For this review, take the finished solid that the model builds, in its own axes (mm). A direction names the side the tool comes from. Give positions to 0.01 mm unless a question says otherwise; leave off trailing zeros. Write each loop counter-clockwise with the first axis right and the second up, starting at its lowest first coordinate (ties: lowest second). Pieces come first, ordered by that corner, then holes. Notation, with made-up numbers: (21, 28) -> (26, 28) arc R9 ccw to (26, 32) -> close; hole circle Ø1 at (9, -30). An arc over 180 degrees is marked (long way). Write item = value, one per line.
```python
from build123d import *

# Parameters (mm, degrees)
BOSS_EXTRUDE1_DEPTH      = 25
BOSS_EXTRUDE1_DEPTH_BACK = 32
SKETCH2_R                = 45
CUT_EXTRUDE1_DEPTH       = 45
CUT_EXTRUDE2_REACH       = 139.165
CUT_EXTRUDE2_END_RADIUS  = 45
SKETCH3_R                = 16
CIRPATTERN1_COUNT        = 6
CHAMFER2_SIZE            = 2
FILLET1_R                = 2


with BuildPart() as part:
    # Sketch1 → Boss-Extrude1 (new, two sides: drawn at the far end of the back side and taken through both)
    with BuildSketch(Plane.XY.offset(-BOSS_EXTRUDE1_DEPTH_BACK)):
        Polygon((0, 61.199128534), (-53, 30.599564267), (-53, -30.599564267), (0, -61.199128534), (53, -30.599564267), (53, 30.599564267), align=None)
    extrude(amount=BOSS_EXTRUDE1_DEPTH + BOSS_EXTRUDE1_DEPTH_BACK)

    # Sketch2 → Cut-Extrude1 (cut)
    with BuildSketch(Plane.XY.offset(25)):
        Circle(SKETCH2_R)
    extrude(amount=-CUT_EXTRUDE1_DEPTH, mode=Mode.SUBTRACT)

    # Cut-Extrude2: up to this cylinder (the profile starts outside it)
    cut_extrude2_end = Plane(origin=(0, 0, 0), z_dir=(0, 0, 1)) * Cylinder(CUT_EXTRUDE2_END_RADIUS, 369.33, mode=Mode.PRIVATE)
    # Sketch3 → Cut-Extrude2 (cut, up to the surface)
    with BuildSketch(Plane(origin=(26.5, -45.899346401, 0), x_dir=(0.8660254037844387, 0.4999999999999999, 0), z_dir=(0.4999999999999999, -0.8660254037844387, 0)), mode=Mode.PRIVATE) as cut_extrude2_sk1:
        Circle(SKETCH3_R)
    cut_extrude2_tool1 = extrude(cut_extrude2_sk1.sketch, amount=-CUT_EXTRUDE2_REACH, mode=Mode.PRIVATE) - cut_extrude2_end
    cut_extrude2 = cut_extrude2_tool1.solids().sort_by_distance((26.5, -45.899346, 0))[0]
    add(cut_extrude2, mode=Mode.SUBTRACT)

    # CirPattern1: Cut-Extrude2 ×6 about axis
    cirpattern1_axis = Axis((0, 0, 25), (0, 0, 1))
    for i in range(1, CIRPATTERN1_COUNT):
        add(cut_extrude2.rotate(cirpattern1_axis, i * 360 / CIRPATTERN1_COUNT), mode=Mode.SUBTRACT)

    # Chamfer2
    chamfer2_edges = [part.edges().sort_by_distance(p)[0] for p in [
        (-45, 0, -20),
    ]]
    chamfer(chamfer2_edges, length=CHAMFER2_SIZE)

    # Fillet1
    fillet1_edges = [part.edges().sort_by_distance(p)[0] for p in [
        (-53, 0, -32),
        (-26.5, -45.899346401, -32),
        (26.5, -45.899346401, -32),
        (53, 0, -32),
        (26.5, 45.899346401, -32),
        (-26.5, 45.899346401, -32),
    ]]
    fillet(fillet1_edges, radius=FILLET1_R)


solid = part.part
```
(1) To check wall thickness, follow probe 1 along Z at (x, y) = (46.75, 0); probe 2 along Z at (x, y) = (15, -9); probe 3 along Y at (x, z) = (39, 9). State the ranges of each line that lie inside material, in increasing order.
Answers below:
probe_1 = -32 to -16, 16 to 25
probe_2 = -32 to -20
probe_3 = -38.68 to -22.45, 22.45 to 38.68
(2) Take a section at B-B (z = 0). Count the separate pieces of the cut face and the enclosed holes in it, plus the area to 3 significant figures.
Answers below:
separate_pieces = 6
enclosed_holes = 0
area = 1,650 mm^2
(3) Take a section at C-C (z = -23). Write out the cut boundary in (x, y).
Answers below:
outline = (-53, -30.6) -> (0, -61.2) -> (53, -30.6) -> (53, 30.6) -> (0, 61.2) -> (-53, 30.6) -> close
(4) Tool access review of faces 1 (the face through (41.569, -17.235, 8.579)), 2 (the face through (-26.59, 45.19, -31.4)): name each direction out of +Z, -Z, +X, -X, +Y, -Y from which nothing blocks a thin tool from reaching the whole face with its end or side.
Answers below:
face_1 = +Z
face_2 = -Z, -X, +Y
(5) Take a section at A-A (y = 0). Write out the cut boundary in (x, z), plus the area to 3 significant figures.
Answers below:
outline = (-53, -30) arc R2 ccw to (-51, -32) -> (51, -32) arc R2 ccw to (53, -30) -> (53, -16) -> (45, -16) -> (45, -18) -> (43, -20) -> (-43, -20) -> (-45, -18) -> (-45, -16) -> (-53, -16) -> close; (-53, 16) -> (-45, 16) -> (-45, 25) -> (-53, 25) -> close; (45, 16) -> (53, 16) -> (53, 25) -> (45, 25) -> close
area = 1,480 mm^2
(6) The part is to be moulded in two halves that separate along X. For faces 3 (the face through (-1, 1, -20)), 4 (the face through (25.84, 45.62, -31.4)), 5 (the face through (-11.61, -49.67, -6.13)), 6 (the face through (-20.24, 49.513, -15.107)), say which applies: released by +X, released by -X, zero draft, split by the parting line, or undercut.
Answers below:
face_3 = undercut
face_4 = released by +X
face_5 = undercut
face_6 = released by -X
(7) For pin 1 (4 mm diameter, centred on x = -9, y = -41, fed in from +Z); pin 2 (5 mm diameter, centred on x = -23, z = 18.5, fed in from +Y); pin 3 (3 mm diameter, centred on y = 15.5, z = -3, fed in from -X); pin 4 (1.5 mm diameter, centred on x = 10, y = 26.5, fed in from +Z), all flat-tipped, find the tip position at first contact; note any pin that passes through.
Answers below:
pin_1 = -19.02
pin_2 = 49.36
pin_3 = -53
pin_4 = -20
